Study the drawing (mm; zero at the part's minimum x, y, z) and answer. A direction names the side the tool comes from. Round coordinates to 2 decimals unless told otherwise and drop trailing zeros. Order: outer loops, then holes, each group sorted by start corner. A loop starts at its lowest first (then second) coordinate and runs counter-clockwise, first axis right, second up. Notation, with made-up numbers: M 41,-39 L 48,-39 A12 ccw 48,-17 Z; hole C 80.5,87 d6. An arc over 180 degrees is marked long. Put each result on its own line as item: value. Start each with the question number.
1. The part is cut by section A-A (y = 19.75). Give the vertices of the cut face in (x, z), then the cut area to 3 significant figures.
2. The part is cut by section C-C (x = 15). Give the vertices of the cut face in (y, z), then the cut area to 3 significant figures.
3. Which of the six approach directions +Z, -Z, +X, -X, +Y, -Y give full straight-line access (tool end or side, diameter ignored) to the marked faces 4 and 5?
4. The part is cut by section D-D (y = 13.25). Give the vertices of the cut face in (x, z), then the cut area to 3 significant figures.
5. The part is cut by section B-B (z = 0.4). Give the vertices of the cut face in (x, y).
6. Each of these flat-tipped pins is pushed along its axis until it touches: pin 1 Ø1.5 at (y, z) = (21.5, 1.5) entering from +X; pin 2 Ø1.5 at (y, z) = (16, 1) entering from -X; pin 3 Ø0.9 at (x, z) = (12.5, 2) entering from +Y. Where does it stop, or does it pass through?
7. Consider line 1 (X direction, y = 3, z = 1.1); line 2 (X direction, y = 3.75, z = 2); line 3 (Y direction, x = 27, z = 1.8). Determine where each line is inside the solid, lowest interval first.
8. The mould has two halves that part along X. Classify the marked faces 1, 2 and 3: +X half, -X half, draft (parallel to the pull), parting line (faces both ways), or undercut.
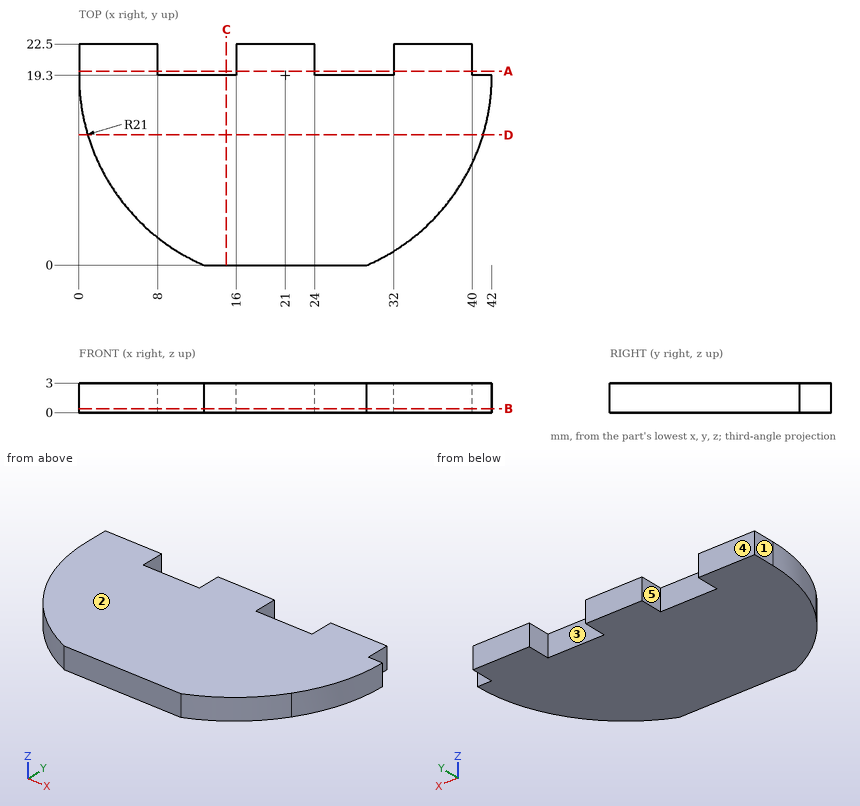
Resolved:
1. outline: M 0,0 L 8,0 L 8,3 L 0,3 Z; M 16,0 L 24,0 L 24,3 L 16,3 Z; M 32,0 L 40,0 L 40,3 L 32,3 Z
1. area: 72.0 mm2
2. outline: M 0,0 L 19.3,0 L 19.3,3 L 0,3 Z
2. area: 57.9 mm2
3. face 4: +Z, -Z, +X, -X, +Y
3. face 5: +Z, -Z, +Y
4. outline: M 0.89,0 L 41.11,0 L 41.11,3 L 0.89,3 Z
4. area: 121 mm2
5. outline: M 0,19.3 A21 ccw 3.43,7.8 A21 ccw 12.72,0 L 29.28,0 A21 ccw 38.57,7.8 A21 ccw 42,19.3 L 40,19.3 L 40,22.5 L 32,22.5 L 32,19.3 L 24,19.3 L 24,22.5 L 16,22.5 L 16,19.3 L 8,19.3 L 8,22.5 L 0,22.5 Z
6. pin 1: x = 40
6. pin 2: x = 0.16
6. pin 3: y = 19.3
7. line 1: 7.76 to 34.24
7. line 2: 6.89 to 35.11
7. line 3: 0 to 19.3
8. face 1: -X half
8. face 2: draft
8. face 3: undercut
